Answer from the drawing. Dimensions are ordinates in mm from the lowest x, y and z of the part. Give positions to 0.01 mm unless a question says otherwise; leave off trailing zeros. Loops run counter-clockwise (first coordinate to the right, second up) from the corner with the lowest first, then second, coordinate; pieces in that order, holes last. Notation, with made-up numbers: (-21.75, 50.25) - (18.25, 50.25) arc R7 cw to (18.25, 55.25) - close; hole circle Ø9 at (22, 6.25). An arc over 180 degrees is marked (long way). One line per question, with ' | ' between items. Start each with the question number.
1. Find the intervals of material crossed by line 1 (X direction, y = 12.5, z = 2.9); line 2 (X direction, y = 12.5, z = 0.35); line 3 (Y direction, x = 133.35, z = 1.8), in increasing order.
2. Section C-C (z = 3.9) is taken. Determine the outline of the cut face in (x, y).
3. Section A-A (x = 133.35) is taken. Determine the outline of the cut face in (y, z).
4. Section B-B (y = 12.5) is taken. Determine the outline of the cut face in (x, z), plus the area to 3 significant figures.
5. Each of these flat-tipped pins is pushed along its axis until it touches: pin 1 (10 mm diameter, centred on x = 99.5, y = 9, fed in from -Z); pin 2 (7.5 mm diameter, centred on x = 133.35, y = 12.5, fed in from -Z). Where does it stop, or does it pass through?
6. Section D-D (x = 92.35) is taken. Determine the outline of the cut face in (y, z).
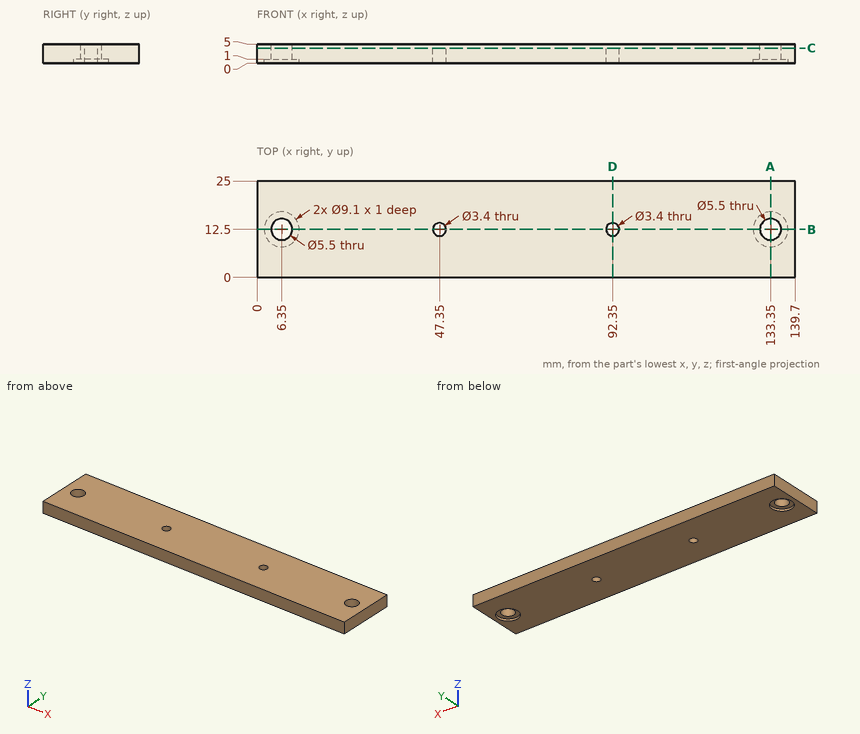
Conclusion:
1) line 1: 0 to 3.6, 9.1 to 45.65, 49.05 to 90.65, 94.05 to 130.6, 136.1 to 139.7 | line 2: 0 to 1.8, 10.9 to 45.65, 49.05 to 90.65, 94.05 to 128.8, 137.9 to 139.7 | line 3: 0 to 9.75, 15.25 to 25
2) outline: (0, 0) - (139.7, 0) - (139.7, 25) - (0, 25) - close; hole circle Ø5.5 at (6.35, 12.5); hole circle Ø3.4 at (47.35, 12.5); hole circle Ø3.4 at (92.35, 12.5); hole circle Ø5.5 at (133.35, 12.5)
3) outline: (0, 0) - (7.95, 0) - (7.95, 1) - (9.75, 1) - (9.75, 5) - (0, 5) - close; (15.25, 1) - (17.05, 1) - (17.05, 0) - (25, 0) - (25, 5) - (15.25, 5) - close
4) outline: (0, 0) - (1.8, 0) - (1.8, 1) - (3.6, 1) - (3.6, 5) - (0, 5) - close; (9.1, 1) - (10.9, 1) - (10.9, 0) - (45.65, 0) - (45.65, 5) - (9.1, 5) - close; (49.05, 0) - (90.65, 0) - (90.65, 5) - (49.05, 5) - close; (94.05, 0) - (128.8, 0) - (128.8, 1) - (130.6, 1) - (130.6, 5) - (94.05, 5) - close; (136.1, 1) - (137.9, 1) - (137.9, 0) - (139.7, 0) - (139.7, 5) - (136.1, 5) - close | area: 602 mm²
5) pin 1: z = 0 | pin 2: z = 1
6) outline: (0, 0) - (10.8, 0) - (10.8, 5) - (0, 5) - close; (14.2, 0) - (25, 0) - (25, 5) - (14.2, 5) - close
